Source: three-view drawing plus pictorial views. Frame: mm from the lowest corner of the part. Round coordinates to 2 decimals unless told otherwise and drop trailing zeros. Loops run counter-clockwise (first coordinate to the right, second up) from the corner with the lowest first, then second, coordinate; pieces in that order, holes last. Notation, with made-up numbers: (-36, -35) -> (-10, -35) arc R22 ccw to (-10, -4) -> close; hole circle Ø11 at (20, 23). An arc over 180 degrees is marked (long way). Answer in a Markdown table with one row per item.
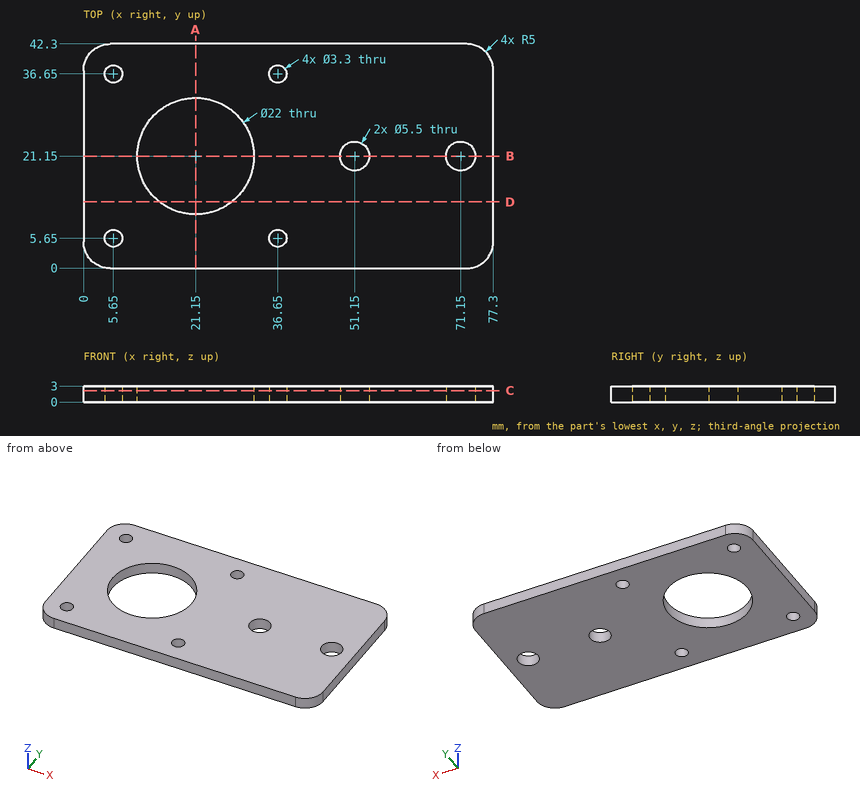
Item 1: Cut plane B-B (y = 21.15). Output: boundary loops of the cut face in (x, z), then the cut area to 3 significant figures.
Answer:
| item | result |
|---|---|
| outline | (0, 0) -> (10.15, 0) -> (10.15, 3) -> (0, 3) -> close; (32.15, 0) -> (48.4, 0) -> (48.4, 3) -> (32.15, 3) -> close; (53.9, 0) -> (68.4, 0) -> (68.4, 3) -> (53.9, 3) -> close; (73.9, 0) -> (77.3, 0) -> (77.3, 3) -> (73.9, 3) -> close |
| area | 133 mm² |
Item 2: Line query: probe 1 along Y at (x, z) = (5.65, 2.25); probe 2 along X at (y, z) = (22.5, 2.5); probe 3 along Y at (x, z) = (21.15, 1.2). Output: solid intervals per line, ascending. Write a range as [from, to].
Answer:
| item | result |
|---|---|
| probe 1 | y = [0, 4], [7.3, 35], [38.3, 42.3] |
| probe 2 | x = [0, 10.23], [32.07, 48.75], [53.55, 68.75], [73.55, 77.3] |
| probe 3 | y = [0, 10.15], [32.15, 42.3] |
Item 3: Cut plane D-D (y = 12.5). Output: boundary loops of the cut face in (x, z), then the cut area to 3 significant figures.
Answer:
| item | result |
|---|---|
| outline | (0, 0) -> (14.35, 0) -> (14.35, 3) -> (0, 3) -> close; (27.95, 0) -> (77.3, 0) -> (77.3, 3) -> (27.95, 3) -> close |
| area | 191 mm² |
Item 4: Cut plane C-C (z = 2.15). Output: boundary loops of the cut face in (x, y).
Answer:
| item | result |
|---|---|
| outline | (0, 5) arc R5 ccw to (5, 0) -> (72.3, 0) arc R5 ccw to (77.3, 5) -> (77.3, 37.3) arc R5 ccw to (72.3, 42.3) -> (5, 42.3) arc R5 ccw to (0, 37.3) -> close; hole circle Ø3.3 at (5.65, 5.65); hole circle Ø3.3 at (5.65, 36.65); hole circle Ø22 at (21.15, 21.15); hole circle Ø3.3 at (36.65, 5.65); hole circle Ø3.3 at (36.65, 36.65); hole circle Ø5.5 at (51.15, 21.15); hole circle Ø5.5 at (71.15, 21.15) |
Item 5: Pin query (flat end, axial travel): pin 1 Ø5 at (x, y) = (69, 29) entering from -Z. Return the tip coordinate at first contact, or that it passes through.
Answer:
| item | result |
|---|---|
| pin 1 | stops at z = 0 |
Item 6: Cut plane A-A (x = 21.15). Output: boundary loops of the cut face in (y, z), then the cut area to 3 significant figures.
Answer:
| item | result |
|---|---|
| outline | (0, 0) -> (10.15, 0) -> (10.15, 3) -> (0, 3) -> close; (32.15, 0) -> (42.3, 0) -> (42.3, 3) -> (32.15, 3) -> close |
| area | 60.9 mm² |
